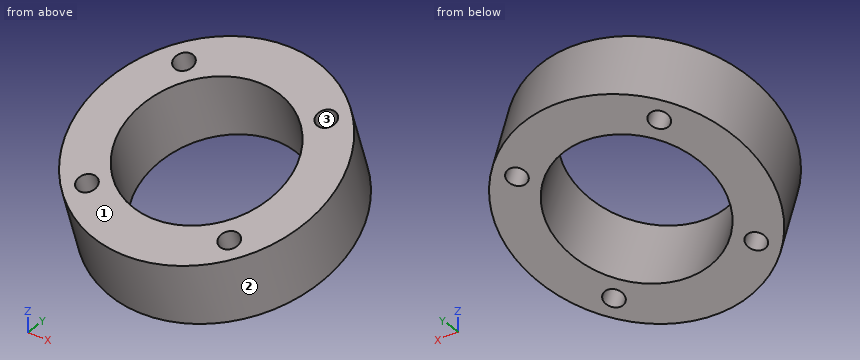
```python
from build123d import *

# Parameters (mm, degrees)
SKETCH1_R               = 31.75
SKETCH1_R_2             = 20.6375
BOSS_EXTRUDE1_DEPTH     = 19.05
F_1_4_20_TAPPED_HOLE1_D = 5.1054


with BuildPart() as part:
    # Sketch1 → Boss-Extrude1 (new body)
    with BuildSketch(Plane(origin=(0, -336.500449063, 1001.043483969), x_dir=(1, 0, 0), z_dir=(0, -0.318629355, 0.947879388))):
        with Locations((0, 892.252904457)):
            Circle(SKETCH1_R)
        with Locations((0, 892.252904457)):
            Circle(SKETCH1_R_2, mode=Mode.SUBTRACT)
    extrude(amount=BOSS_EXTRUDE1_DEPTH)

    # 1/4-20 Tapped Hole1 (through all)
    with Locations(Plane(origin=(0, -336.500449063, 1001.043483969), x_dir=(-1, 0, 0), z_dir=(0, 0.318629355, -0.947879388))):
        with Locations((18.52177825, 910.774682707), (-18.52177825, 910.774682707), (-18.52177825, 873.731126207), (18.52177825, 873.731126207)):
            Hole(F_1_4_20_TAPPED_HOLE1_D / 2)


solid = part.part
```
CAD build for the part. Positions are in the model's coordinates, mm. Face numbers are marked on the shaded views. Give positions to 0.01 mm unless a question says otherwise; leave off trailing zeros. Loops run counter-clockwise (first coordinate to the right, second up) from the corner with the lowest first, then second, coordinate; pieces in that order, holes last. Notation, with made-up numbers: M 46.5,11 L 93.5,11 A23 ccw 93.5,33 Z; hole C 23.5,80.5 d8. An arc over 180 degrees is marked long. Use one line per item in the form item = value.
Item 1: Drill centre lines: probe 1 along Y at (x, z) = (19, 1283.5); probe 2 along X at (y, z) = (490, 1291.5); probe 3 along Y at (x, z) = (-16.5, 1282.5). Where is each one in solid material? Low to high. Write a range as from..to.
Determined:
probe_1 = 483.03..487.68, 492.97..501.37
probe_2 = -27.26..-19.75, -17.3..-12.68, 12.68..17.3, 19.75..27.26
probe_3 = 481.59..489.02, 492.31..497.13
Item 2: Flat gauge pins, fed straight in: pin 1 (3 mm diameter, centred on x = 20, y = 493, fed in from -Z); pin 2 (2 mm diameter, centred on y = 484.5, z = 1284.5, fed in from -X); pin 3 (10 mm diameter, centred on y = 531, z = 1303.5, fed in from -X). Where does each tip first touch, or does it go through?
Determined:
pin_1 = 1279.52
pin_2 = -22.17
pin_3 = -23.45
Item 3: Slice it at B-B (x = -19.5). List the corners of the cut face in (y, z), plus the area to 3 significant figures.
Determined:
outline = M 479.43,1295.41 L 485.5,1277.36 L 489.46,1278.69 L 483.39,1296.75 Z; M 487.86,1298.25 L 493.93,1280.19 L 502.84,1283.19 L 496.77,1301.25 Z; M 509.58,1305.55 L 515.65,1287.49 L 524.57,1290.49 L 518.5,1308.55 Z; M 522.97,1310.05 L 529.04,1291.99 L 533,1293.33 L 526.93,1311.38 Z
area = 518 mm2
Item 4: Two-plate mould, pull along Y, no slides. Class the marked faces 1, 2 and 3: pulls with the +Y half, pulls with the -Y half, needs draft (parallel to the pull), parting line crosses it, or undercut.
Determined:
face_1 = pulls with the -Y half
face_2 = parting line crosses it
face_3 = undercut
Item 5: Slice it at C-C (x = -11). List the corners of the cut face in (y, z), plus the area to 3 significant figures.
Determined:
outline = M 474.95,1293.91 L 481.02,1275.85 L 492.7,1279.78 L 486.63,1297.83 Z; M 519.73,1308.96 L 525.8,1290.91 L 537.48,1294.83 L 531.41,1312.89 Z
area = 469 mm2
Item 6: Slice it at A-A (x = -1.5). List the corners of the cut face in (y, z), plus the area to 3 significant figures.
Determined:
outline = M 473.12,1293.29 L 479.19,1275.24 L 489.74,1278.78 L 483.67,1296.84 Z; M 522.69,1309.96 L 528.76,1291.9 L 539.31,1295.45 L 533.24,1313.5 Z
area = 424 mm2
Item 7: Slice it at D-D (y = 524). Count the separate pieces of the cut face and the enclosed holes in it, plus the area to 3 significant figures.
Determined:
separate_pieces = 1
enclosed_holes = 2
area = 601 mm2
